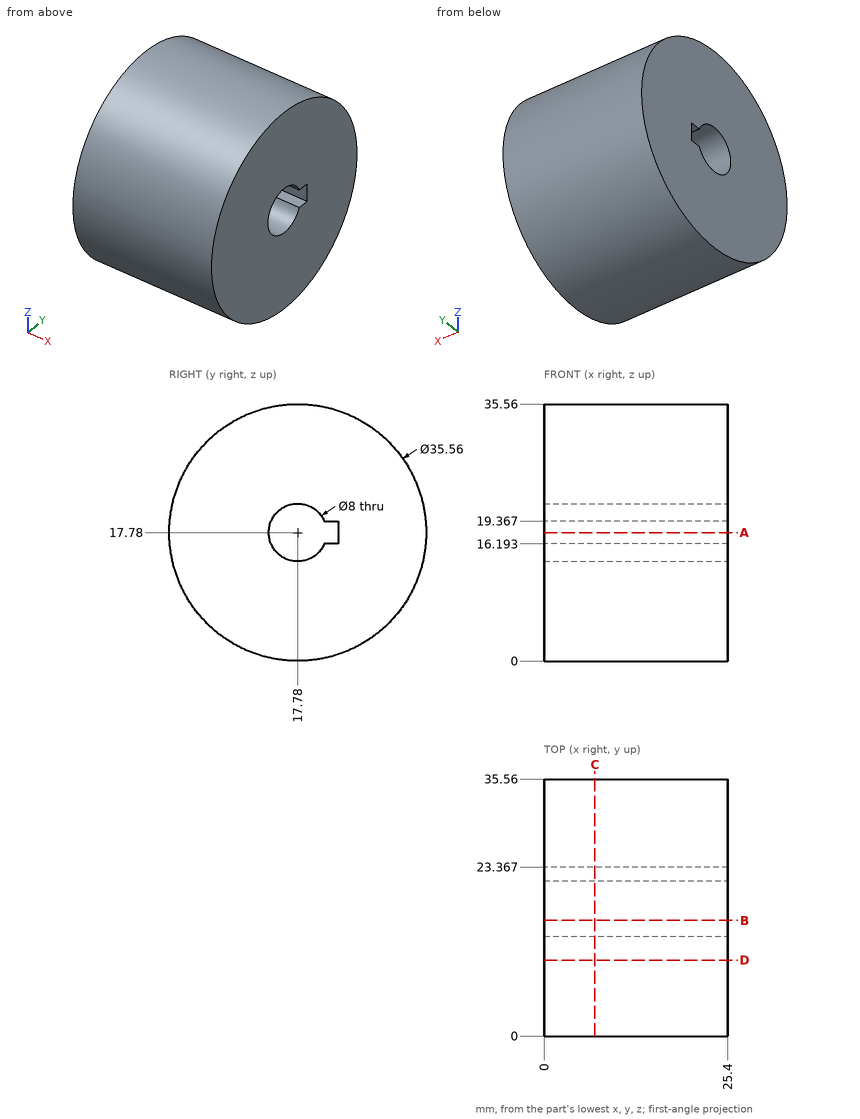
The drawing under review shows one solid part. Ordinate dimensions are in mm from its lowest x, y, z. Coordinates: 2 decimals unless noted, no trailing zeros. Write each loop counter-clockwise with the first axis right and the second up, starting at its lowest first coordinate (ties: lowest second). Pieces come first, ordered by that corner, then holes. Notation, with made-up numbers: (81.5, 44) - (109.5, 44) arc R16 cw to (109.5, 49) - close; hole circle Ø2 at (-27.75, 23.25). An arc over 180 degrees is marked (long way). Answer as CSV lines item,"result".
(1) We need section A-A (z = 17.78). Give the boundary of the cut face in (x, y).
Data:
outline,"(0, 0) - (25.4, 0) - (25.4, 13.78) - (0, 13.78) - close; (0, 23.37) - (25.4, 23.37) - (25.4, 35.56) - (0, 35.56) - close"
(2) For line 1 along Z through (x, y) = (8.5, 17.78); line 2 along Y through (x, z) = (16.5, 17.78); line 3 along Z through (x, y) = (19.75, 19.5) (1 decimal), list the stretches that pass through material, from the lowest coordinate up. Write a range as [from, to].
Data:
line 1,"z = [0, 13.78], [21.78, 35.56]"
line 2,"y = [0, 13.78], [23.37, 35.56]"
line 3,"z = [0.1, 14.2], [21.4, 35.5]"
(3) We need section D-D (y = 10.5). Give the boundary of the cut face in (x, z), plus the area to 3 significant figures.
Data:
outline,"(0, 1.56) - (25.4, 1.56) - (25.4, 34) - (0, 34) - close"
area,"824 mm2"
(4) Clearance check with flat-ended pins moving along their axes: pin 1 Ø4 at (x, z) = (20.5, 17.5) entering from +Y; pin 2 Ø4 at (x, z) = (7.5, 4) entering from +Y; pin 3 Ø5 at (x, z) = (5.5, 12) entering from +Y (1 decimal); pin 4 Ø8 at (x, y) = (16.5, 4) entering from -Z. State where each tip first meets the part, or that it passes through.
Data:
pin 1,"stops at y = 35.56"
pin 2,"stops at y = 31.1"
pin 3,"stops at y = 35.3"
pin 4,"stops at z = 2.93"
(5) We need section C-C (x = 7). Give the boundary of the cut face in (y, z).
Data:
outline,"circle Ø35.56 at (17.78, 17.78); hole (21.45, 16.19) - (23.37, 16.19) - (23.37, 19.37) - (21.45, 19.37) arc R4 ccw (long way) to start"
(6) We need section B-B (y = 16). Give the boundary of the cut face in (x, z), plus the area to 3 significant figures.
Data:
outline,"(0, 0.09) - (25.4, 0.09) - (25.4, 14.2) - (0, 14.2) - close; (0, 21.36) - (25.4, 21.36) - (25.4, 35.47) - (0, 35.47) - close"
area,"717 mm2"
